from build123d import *

# Parameters (mm, degrees)
F0_R     = 4
F0_R_2   = 1.5
F1_DEPTH = 15
F3_DEPTH = 1.5


with BuildPart() as f1:
    # F0 (on Right) → F1 (new body)
    with BuildSketch(Plane.YZ):
        Circle(F0_R)
        Circle(F0_R_2, mode=Mode.SUBTRACT)
    extrude(amount=F1_DEPTH)

    # F2 (on Front) → F3 (join, symmetric)
    with BuildSketch(Plane.XZ):
        with BuildLine():
            Line((14.70626425, -3), (0, -3))
            Line((0, -3), (4.5474985961, -11.9707668002))
            ThreePointArc((4.5474985961, -11.9707668002), (8.9263863781, -14.1716151823), (12.3194694103, -10.6353206038))
            Line((12.3194694103, -10.6353206038), (10.7860491436, -9.75))
            ThreePointArc((10.7860491436, -9.75), (5.90120114, -9), (10.7860491436, -8.25))
            Line((10.7860491436, -8.25), (13.3405016736, -6.7751861441))
            Line((13.3405016736, -6.7751861441), (14.70626425, -3))
        make_face()
    extrude(amount=F3_DEPTH, both=True)

    # F5: F1 across plane


with BuildPart() as f1_1:
    add(f1.part)
    add(f1.part.mirror(Plane.XY.offset(-9)))


solid = f1_1.part
Design review of the part built by this model. Coordinates are the model's own, in mm. A direction names the side the tool comes from. Round coordinates to 2 decimals unless told otherwise and drop trailing zeros. Write each loop counter-clockwise with the first axis right and the second up, starting at its lowest first coordinate (ties: lowest second). Pieces come first, ordered by that corner, then holes. Notation, with made-up numbers: (30.25, 8.25) - (42.25, 8.25) arc R26 cw to (42.25, 32.25) - close; hole circle Ø11 at (89.5, 85). An arc over 180 degrees is marked (long way). Return JSON: item names as keys, results as strings. Group by question number.
Item 1: Machinability: for faces 3 (the face through (7.395, -0.195, -19.487)), 4 (the face through (5.7, -1.5, -9.1)), 5 (the face through (5.7, 1.5, -9.1)), which of the approach directions +Z, -Z, +X, -X, +Y, -Y give a long, thin tool a straight path to every point of the face, cutting with its end or side? Answer none if there is none.
Item 2: The part is to be moulded in two halves that separate along Z. For faces 1 (the face through (15, 0, -16)), 2 (the face through (12.05, -0.02, -7.52)), say which applies: pulls with the +Z half, pulls with the -Z half, needs draft (parallel to the pull), parting line crosses it, or undercut.
Item 3: We need section B-B on z = 0. Write out the cut boundary in (x, y).
Item 4: We need section C-C on y = 0. Write out the cut boundary in (x, z), and give its area (3 significant figures).
Item 5: Insertion check: P1, Ø1.5, axis at x = 13.5, z = -7.5, coming from the +Y side; P2, Ø6, axis at x = 4.5, z = -14, coming from the +Y side; P3, Ø1, axis at x = 13.5, z = -14.5, coming from the +Y side; P4, Ø8, axis at x = 3.5, z = -16.5, coming from the +Y side. Each pin has a flat end and moves straight along its axis. Give the tip position at first contact, or say it passes through.
Item 6: We need section D-D on x = 4.25. Write out the cut boundary in (y, z).
Item 7: We need section A-A on x = 1.25. Write out the cut boundary in (y, z).
Item 8: For probe 1 along Z at (x, y) = (2.25, 0.5); probe 2 along Z at (x, y) = (7.5, 0); probe 3 along Y at (x, z) = (13.75, -18.75), list the stretches that pass through material, from the lowest coordinate up. Write a range as [from, to].
Model answer:
{
 "1": {"face 3": "+X, -X", "face 4": "+X, -X, -Y", "face 5": "+X, -X, +Y"},
 "2": {"face 1": "needs draft", "face 2": "undercut"},
 "3": {"outline": "(0, -4) - (15, -4) - (15, -1.5) - (0, -1.5) - close; (0, 1.5) - (15, 1.5) - (15, 4) - (0, 4) - close"},
 "4": {"outline": "(0, -22) - (15, -22) - (15, -19.5) - (0, -19.5) - close; (0, -16.5) - (15, -16.5) - (15, -14) - (14.34, -14) - (13.34, -11.22) - (10.79, -9.75) arc R2.5 cw (long way) to (10.79, -8.25) - (13.34, -6.78) - (14.34, -4) - (15, -4) - (15, -1.5) - (0, -1.5) - (0, -4) - (0.51, -4) - (3.04, -9) - (0.51, -14) - (0, -14) - close; (0, 1.5) - (15, 1.5) - (15, 4) - (0, 4) - close", "area": "241 mm²"},
 "5": {"P1": "stops at y = 1.5", "P2": "stops at y = 3.87", "P3": "stops at y = 2.65", "P4": "stops at y = 4"},
 "6": {"outline": "(-1.5, -14.29) arc R4 ccw (long way) to (1.5, -14.29) - (1.5, -3.71) arc R4 ccw (long way) to (-1.5, -3.71) - close; hole circle Ø3 at (0, -18); hole circle Ø3 at (0, 0)"},
 "7": {"outline": "(-1.5, -14.29) arc R4 ccw (long way) to (1.5, -14.29) - (1.5, -12.53) - (-1.5, -12.53) - close; (-1.5, -5.47) - (1.5, -5.47) - (1.5, -3.71) arc R4 ccw (long way) to (-1.5, -3.71) - close; hole circle Ø3 at (0, -18); hole circle Ø3 at (0, 0)"},
 "8": {"probe 1": "z = [-21.97, -19.41], [-16.59, -10.56], [-7.44, -1.41], [1.41, 3.97]", "probe 2": "z = [-22, -19.5], [-16.5, -11.33], [-6.67, -1.5], [1.5, 4]", "probe 3": "y = [-3.93, -1.3], [1.3, 3.93]"}
}
